from build123d import *

# Parameters (mm, degrees)
SKETCH_1_R               = 3
SKETCH_1_R_2             = 1.65
EXTRUDE_1_DEPTH          = 4
CUT_EXTRUDE_2_DEPTH      = 6.830951895
PATTERN_CIRCULAR_1_COUNT = 9
SKETCH_2_R               = 3
EXTRUDE_2_DEPTH          = 0.8
EXTRUDE_START            = 0.8
EXTRUDE_3_DEPTH          = 1.5
EXTRUDE_START_2          = -4
SKETCH_2_4_R             = 3
EXTRUDE_4_DEPTH          = 4
CUT_EXTRUDE_3_DEPTH      = 3.8


with BuildPart() as part:
    # 草图1 → 凸台-拉伸1 (new body)
    with BuildSketch(Plane.XY):
        Circle(SKETCH_1_R)
        Circle(SKETCH_1_R_2, mode=Mode.SUBTRACT)
    extrude(amount=EXTRUDE_1_DEPTH)

    # 草图1<3> → 切除-拉伸2 (cut, through all)
    with BuildSketch(Plane.XY):
        with BuildLine():
            Line((1.583201231, 0.595370355), (1.54440693, 0.580781573))
            ThreePointArc((1.54440693, 0.580781573), (1.623387112, 0.295151288), (1.65, 0))
            ThreePointArc((1.65, 0), (1.623387112, -0.295151288), (1.54440693, -0.580781573))
            Line((1.54440693, -0.580781573), (1.583201231, -0.595370355))
            add(Edge.make_bspline(
                [(1.583201231, -0.595370355), (1.595268082, -0.599908151), (1.629927649, -0.609960022), (1.698544644, -0.618780808), (1.810680065, -0.617601716), (1.954246735, -0.59352555), (2.132298369, -0.536822163), (2.302941373, -0.452472776), (2.42578745, -0.372108406), (2.505673341, -0.310927028), (2.533645284, -0.288342805)],
                knots=[0, 0, 0, 0, 0, 0.005604068, 0.015718248, 0.029959916, 0.048733667, 0.068727063, 0.096888892, 0.112551479, 0.112551479, 0.112551479, 0.112551479, 0.112551479], degree=4))
            ThreePointArc((2.533645284, -0.288342805), (2.545908038, -0.144403125), (2.55, 0))
            ThreePointArc((2.55, 0), (2.545908038, 0.144403125), (2.533645284, 0.288342805))
            add(Edge.make_bspline(
                [(1.583201231, 0.595370355), (1.595268082, 0.599908151), (1.629927649, 0.609960022), (1.698544644, 0.618780808), (1.810680065, 0.617601716), (1.954246735, 0.59352555), (2.132298369, 0.536822163), (2.302941373, 0.452472776), (2.42578745, 0.372108406), (2.505673341, 0.310927028), (2.533645284, 0.288342805)],
                knots=[0, 0, 0, 0, 0, 0.005604068, 0.015718248, 0.029959916, 0.048733667, 0.068727063, 0.096888892, 0.112551479, 0.112551479, 0.112551479, 0.112551479, 0.112551479], degree=4))
        make_face()
    cut_extrude_2 = extrude(amount=CUT_EXTRUDE_2_DEPTH, mode=Mode.SUBTRACT)

    # 阵列(圆周)1: 切除-拉伸2 ×9 about axis
    pattern_circular_1_axis = Axis((0, 0, 4), (0, 0, 1))
    for i in range(1, PATTERN_CIRCULAR_1_COUNT):
        add(cut_extrude_2.rotate(pattern_circular_1_axis, i * 360 / PATTERN_CIRCULAR_1_COUNT), mode=Mode.SUBTRACT)

    # 草图2 → 凸台-拉伸2 (add)
    with BuildSketch(Plane.XY.offset(4)):
        Circle(SKETCH_2_R)
    extrude(amount=EXTRUDE_2_DEPTH)

    # 草图2<3> → 凸台-拉伸3 (add)
    with BuildSketch(Plane.XY.offset(4).offset(EXTRUDE_START)):
        Polygon((0.635085296, 1.1), (-0.635085296, 1.1), (-1.270170592, 0), (-0.635085296, -1.1), (0.635085296, -1.1), (1.270170592, 0), align=None)
    extrude(amount=EXTRUDE_3_DEPTH)

    # 草图2<4> → 凸台-拉伸4 (add)
    with BuildSketch(Plane.XY.offset(4).offset(EXTRUDE_START_2)):
        Circle(SKETCH_2_4_R)
    extrude(amount=EXTRUDE_4_DEPTH)

    # 草图3 → 切除-拉伸3 (cut)
    with BuildSketch(Plane(origin=(0, 0, 0), x_dir=(-1, 0, 0), z_dir=(0, 0, -1))):
        with BuildLine():
            Line((1.1, -1.092016483), (1.1, 1.092016483))
            ThreePointArc((1.1, 1.092016483), (-1.55, 0), (1.1, -1.092016483))
        make_face()
    extrude(amount=-CUT_EXTRUDE_3_DEPTH, mode=Mode.SUBTRACT)


solid = part.part
Check sheet for the modelled part. Datum: model origin and axes. Units: mm. A direction names the side the tool comes from. Give positions to 0.01 mm unless a question says otherwise; leave off trailing zeros. Order: outer loops, then holes, each group sorted by start corner. A loop starts at its lowest first (then second) coordinate and runs counter-clockwise, first axis right, second up. Notation, with made-up numbers: (-12.75, 15.25) - (21.25, 15.25) arc R17 cw to (21.25, 45.25) - close; hole circle Ø7 at (20.25, 2.25). An arc over 180 degrees is marked (long way). Answer as CSV lines item,"result".
1. Scan lines: probe 1 along Y at (x, z) = (0, 2.3); probe 2 along Z at (x, y) = (1.5, 0); probe 3 along Z at (x, y) = (2.2, -1.3). Record each from-to range of solid material in increasing order. Write a range as from..to.
Result sheet:
probe 1,"-3..-1.55, 1.55..3"
probe 2,"3.8..4.8"
probe 3,"0..4.8"
2. Section check B-B (z = 5.75). Record the boundary of the cut face in (x, y).
Result sheet:
outline,"(-1.27, 0) - (-0.64, -1.1) - (0.64, -1.1) - (1.27, 0) - (0.64, 1.1) - (-0.64, 1.1) - close"
3. Section check A-A (x = 0). Record the boundary of the cut face in (y, z), then the cut area to 3 significant figures.
Result sheet:
outline,"(-3, 0) - (-1.55, 0) - (-1.55, 3.8) - (1.55, 3.8) - (1.55, 0) - (3, 0) - (3, 4.8) - (1.1, 4.8) - (1.1, 6.3) - (-1.1, 6.3) - (-1.1, 4.8) - (-3, 4.8) - close"
area,"20.3 mm²"
4. Go/stop test with flat-tipped pins: P1, Ø3, axis at x = 1.5, y = -2.5, coming from the +Z side; P2, Ø0.6, axis at x = 0.5, z = 5.5, coming from the -Y side; P3, Ø0.6, axis at x = 0, z = 6, coming from the +Y side. Record where each tip stops, or that it passes through.
Result sheet:
P1,"z = 4.8"
P2,"y = -1.1"
P3,"y = 1.1"
5. Section check C-C (z = 2). Record the boundary of the cut face in (x, y), then the cut area to 3 significant figures.
Result sheet:
outline,"circle Ø6 at (0, 0); hole (-1.1, -1.09) arc R1.55 ccw (long way) to (-1.1, 1.09) - close"
area,"21.4 mm²"
6. Mould release check, pull along Y, two halves, no side actions. Record for faces 6 (the face through (0, 0, 6.3)), 7 (the face through (0, -1.1, 6)), 8 (the face through (-1.1, 0, 2)): released by +Y, released by -Y, zero draft, split by the parting line, or undercut.
Result sheet:
face 6,"zero draft"
face 7,"released by -Y"
face 8,"undercut"
7. Section check D-D (y = 2). Record the boundary of the cut face in (x, z).
Result sheet:
outline,"(-2.24, 0) - (2.24, 0) - (2.24, 4.8) - (-2.24, 4.8) - close"
8. Tool access check on faces 1 (the face through (-0.96, -0.54, 5.54)), 2 (the face through (-0.948, 0.558, 5.54)), 3 (the face through (0.948, -0.558, 5.54)), 4 (the face through (0, -1.3, 4.8)), 5 (the face through (0.96, 0.54, 5.54)). Record the directions out of +Z, -Z, +X, -X, +Y, -Y that give a thin tool (end or side, any length) a straight path to the whole face; none if there is none.
Result sheet:
face 1,"+Z, -X, -Y"
face 2,"+Z, -X, +Y"
face 3,"+Z, +X, -Y"
face 4,"+Z"
face 5,"+Z, +X, +Y"
